Work out the finished part from the listing and answer in its coordinate system (mm). A direction names the side the tool comes from. Coordinates: 2 decimals unless noted, no trailing zeros. Order: outer loops, then holes, each group sorted by start corner. A loop starts at its lowest first (then second) coordinate and runs counter-clockwise, first axis right, second up.
1. Flat-ended cylindrical pins translate along their axes: pin 1 Ø5 at (y, z) = (42.5, -30) entering from -X; pin 2 Ø3 at (x, y) = (-35.5, 48.5) entering from -Z. Find the tip coordinate at first contact, or state that the pin passes through.
2. The part is cut by section D-D, the plane z = -9. Give the vertices of the cut face in (x, y), then the cut area to 3 significant figures.
3. The part is cut by section A-A, the plane x = -14. Give the vertices of the cut face in (y, z), then the cut area to 3 significant figures.
4. A tool of negligible diameter and unlimited length cuts with its end or side. For faces 1 (the flat face through (-34, 38, -12.7)), 2 (the flat face through (-23, 29, 0)), 3 (the flat face through (-32.2, 6.3, -6.3)), from which of +Z, -Z, +X, -X, +Y, -Y can it reach the whole face along a straight path? Write none if from no direction.
5. Determine the mould class of faces 4 (the flat face through (-3, 38, -38.1)), 5 (the cylindrical face through (-13.26, 29.8, -6.44)), 6 (the flat face through (0, 38, -19)), 7 (the flat face through (-6.35, 38, -26)) for opening direction X: +X half, -X half, draft (parallel to the pull), parting line (faces both ways), or undercut.
6. The part is cut by section C-C, the plane y = 71. Give the vertices of the cut face in (x, z), then the cut area to 3 significant figures.
7. Find the intervals of material crossed by probe 1 along Y at (x, z) = (-12, -8.5); probe 2 along X at (y, z) = (57, -10.5); probe 3 along Z at (x, y) = (-12, 32.5), in increasing order.
8. The part is cut by section B-B, the plane z = -25.4. Give the vertices of the cut face in (x, y), then the cut area to 3 significant figures.
```python
from build123d import *

# Parameters (mm, degrees)
BOSS_EXTRUDE1_DEPTH = 76.2
SKETCH4_R           = 2.0574
CUT_EXTRUDE3_DEPTH  = 7.35
SKETCH3_R           = 13.589
SKETCH3_R_2         = 2.54
CUT_EXTRUDE2_DEPTH  = 13.7
CUT_EXTRUDE4_DEPTH  = 12.7


with BuildPart() as part:
    # Sketch1 → Boss-Extrude1 (new body)
    with BuildSketch(Plane(origin=(0, 0, 0), x_dir=(1, 0, 0), z_dir=(0, 1, 0))):
        Polygon((-44.45, 12.7), (-44.45, 0), (0, 0), (0, 38.1), (-6.35, 38.1), (-6.35, 12.7), align=None)
    extrude(amount=BOSS_EXTRUDE1_DEPTH)

    # Sketch4 → Cut-Extrude3 (cut, through all)
    with BuildSketch(Plane.ZY.offset(6.35)):
        with Locations((-25.4, 22.7838)):
            Circle(SKETCH4_R)
        with Locations((-25.4, 34.036)):
            Circle(SKETCH4_R)
    extrude(amount=-CUT_EXTRUDE3_DEPTH, mode=Mode.SUBTRACT)

    # Sketch3 → Cut-Extrude2 (cut, through all)
    with BuildSketch(Plane(origin=(0, 0, -12.7), x_dir=(-1, 0, 0), z_dir=(0, 0, -1))):
        with Locations((19.939, 46.3296)):
            Circle(SKETCH3_R)
        with Locations((35.179, 57.7596)):
            Circle(SKETCH3_R_2)
        with Locations((13.589, 65.3796)):
            Circle(SKETCH3_R_2)
        with Locations((13.589, 27.2796)):
            Circle(SKETCH3_R_2)
        with Locations((35.179, 34.8996)):
            Circle(SKETCH3_R_2)
    extrude(amount=-CUT_EXTRUDE2_DEPTH, mode=Mode.SUBTRACT)

    # Sketch6 → Cut-Extrude4 (cut)
    with BuildSketch(Plane.XZ):
        Polygon((-47.891108231, 6.866314065), (10.481478335, -42.114101793), (8.522261701, -44.449005256), (-49.850324865, 4.531410602), align=None)
    extrude(amount=-CUT_EXTRUDE4_DEPTH, mode=Mode.SUBTRACT)


solid = part.part
```
Geometry says:
1. pin 1: stops at x = -6.35
1. pin 2: stops at z = -12.7
2. outline: (-44.45, 0) - (-33.72, 0) - (-33.72, 12.7) - (-28.98, 12.7) - (-28.98, 0) - (0, 0) - (0, 76.2) - (-44.45, 76.2) - close; hole circle Ø5.08 at (-35.18, 34.9); hole circle Ø5.08 at (-35.18, 57.76); hole circle Ø27.18 at (-19.94, 46.33); hole circle Ø5.08 at (-13.59, 27.28); hole circle Ø5.08 at (-13.59, 65.38)
2. area: 2,670 mm2
3. outline: (0, -12.7) - (24.77, -12.7) - (24.77, 0) - (0, 0) - close; (29.79, -12.7) - (34.11, -12.7) - (34.11, 0) - (29.79, 0) - close; (58.55, -12.7) - (62.87, -12.7) - (62.87, 0) - (58.55, 0) - close; (67.89, -12.7) - (76.2, -12.7) - (76.2, 0) - (67.89, 0) - close
3. area: 530 mm2
4. face 1: -Z, -X, +Y, -Y
4. face 2: +Z, +X, -X, +Y, -Y
4. face 3: -Y
5. face 4: draft
5. face 5: undercut
5. face 6: +X half
5. face 7: -X half
6. outline: (-44.45, -12.7) - (-6.35, -12.7) - (-6.35, -38.1) - (0, -38.1) - (0, 0) - (-44.45, 0) - close
6. area: 726 mm2
7. probe 1: y = 0 to 25.3, 29.26 to 35.3, 57.36 to 63.4, 67.36 to 76.2
7. probe 2: x = -44.45 to -37.6, -32.76 to -28.35, -11.52 to 0
7. probe 3: z = -12.7 to 0
8. outline: (-6.35, 0) - (0, 0) - (0, 20.73) - (-6.35, 20.73) - close; (-6.35, 24.84) - (0, 24.84) - (0, 31.98) - (-6.35, 31.98) - close; (-6.35, 36.09) - (0, 36.09) - (0, 76.2) - (-6.35, 76.2) - close
8. area: 432 mm2
